Autodesk Inventor part; units mm, degrees
ref_plane "YZ Plane" through (0, 0, 0) normal (1, 0, 0) x (0, 1, 0)
ref_plane "XZ Plane" through (0, 0, 0) normal (0, 1, 0) x (-1, 0, 0)
ref_plane "XY Plane" through (0, 0, 0) normal (0, 0, 1) x (1, 0, 0)
sketch "Sketch1" plane through (0, 0, 0) normal (0, 0, 1) x (1, 0, 0)
  line L0 (-25, -35) -> (25, -35)
  line L1 (30, -30) -> (30, 30)
  line L2 (25, 35) -> (-25, 35)
  line L3 (-30, 30) -> (-30, -30)
  line L4 (-30, -35) -> (30, 35) construction
  line L5 (30, -35) -> (-30, 35) construction
  arc A0 (-25, 35) -> (-30, 30) centre (-25, 30) ccw
  arc A1 (30, 30) -> (25, 35) centre (25, 30) ccw
  arc A2 (25, -35) -> (30, -30) centre (25, -30) ccw
  arc A3 (-30, -30) -> (-25, -35) centre (-25, -30) ccw
  point P0 (0, 0)
  dimension "d0" = 60
  dimension "d1" = 70
  dimension "d4" = 5
extrude "Extrusion1" add sketch "Sketch1" along normal blind 5
sketch "Sketch2" plane through (0, 0, 5) normal (0, 0, 1) x (1, 0, 0)
  line L0 (-22.5, -30.0466) -> (22.5, -30.0466) construction
  line L1 (22.5, -30.0466) -> (22.5, -10.0466) construction
  line L2 (22.5, -10.0466) -> (-22.5, -10.0466) construction
  line L3 (-22.5, -10.0466) -> (-22.5, -30.0466) construction
  line L4 (-22.5, -30.0466) -> (22.5, -10.0466) construction
  line L5 (22.5, -30.0466) -> (-22.5, -10.0466) construction
  point P0 (0, 0)
  point P1 (0, -20.0466)
  point P2 (0, -20.0466)
  dimension "d5" = 45
  dimension "d6" = 20.0466
  dimension "d7" = 20
hole "Hole1" at (22.5, -10.0466, 5) at (22.5, -30.0466, 5) at (-22.5, -30.0466, 5) direction (0, 0, -1) diameter 5.5 depth 8 tip angle 118
sketch "Sketch3" plane through (0, 0, 5) normal (0, 0, 1) x (1, 0, 0)
  line L0 (-2.5, 0) -> (2.5, 0)
  line L1 (2.5, 0) -> (2.5, 20)
  line L2 (2.5, 20) -> (-2.5, 20)
  line L3 (-2.5, 20) -> (-2.5, 0)
  line L4 (-2.5, 0) -> (2.5, 20) construction
  line L5 (2.5, 0) -> (-2.5, 20) construction
  point P0 (0, 0)
  point P1 (0, 10)
  point P2 (0, 10)
  point P3 (0, 0)
  point P4 (0, 10)
  dimension "d15" = 5
  dimension "d16" = 20
  dimension "d17" = 10
extrude "Extrusion2" cut sketch "Sketch3" against normal blind 5
sketch "Sketch4" plane through (0, 0, 5) normal (0, 0, 1) x (1, 0, 0)
  line L0 (-2.5, 20) -> (2.5, 20)
  line L1 (2.5, 0) -> (-2.5, 0)
  point P0 (0, 0)
  point P1 (0, 28)
  point P2 (0, -8)
  point P3 (0, 0)
  dimension "d20" = 8
  dimension "d21" = 8
hole "Hole2" at (0, 28, 5) at (0, -8, 5) direction (0, 0, -1) diameter 4.5 depth 8 tip angle 118
sketch "Sketch5" plane through (0, 0, 5) normal (0, 0, 1) x (1, 0, 0)
  line L0 (2.5, 0) -> (-2.5, 0)
  line L1 (-20, -25) -> (-10, -25)
  line L2 (-10, -25) -> (-10, -20)
  line L3 (-10, -20) -> (-20, -20)
  line L4 (-20, -20) -> (-20, -25)
  line L5 (-20, -25) -> (-10, -20) construction
  line L6 (-10, -25) -> (-20, -20) construction
  line L7 (-25, -35) -> (25, -35)
  line L8 (-30, 30) -> (-30, -30)
  point P0 (0, 0)
  point P1 (0, 0)
  point P2 (-15, -22.5)
  dimension "d34" = 10
  dimension "d35" = 5
  dimension "d36" = 10
  dimension "d37" = 30
  dimension "d38" = 10
extrude "Extrusion3" cut sketch "Sketch5" against normal blind 5
equation "\"d38\" = -0.5 * d34 + 0.5 * d37"
properties part number "Belt_Holder1" material "Polycarbonate, Clear"
Could you check a few things on this model? Use its own coordinates, in mm. A direction names the side the tool comes from. Coordinates: 2 decimals unless noted, no trailing zeros. Write each loop counter-clockwise with the first axis right and the second up, starting at its lowest first coordinate (ties: lowest second). Pieces come first, ordered by that corner, then holes. Notation, with made-up numbers: (1, -10) -> (49, -10) arc R25 ccw to (49, 11) -> close; hole circle Ø9 at (10.25, 77.5). An arc over 180 degrees is marked (long way). One line per question, with ' | ' between items. Start each with the question number.
1. If we section it at D-D (z = 2.1): Please give me the cut outline in (x, y), and give its area (3 significant figures).
2. If we section it at B-B (y = 11): Please give me the cut outline in (x, z).
3. Please list where these lines run through material, in increasing order: line 1 along Y through (x, z) = (0, 1.3); line 2 along Y through (x, z) = (22.5, 2.35); line 3 along X through (y, z) = (3, 2.95).
4. Thinking about a two-plate mould opening in X: for faces 1 (the face through (28, 34, 2)), 2 (the face through (-29, 33, 2)), 3 (the face through (19.773, -9.689, 2.465)), which applies, pulls with the +X half, pulls with the -X half, needs draft (parallel to the pull), parting line crosses it, or undercut?
5. If we section it at A-A (x = 0): Please give me the cut outline in (y, z).
6. For faces 4 (the face through (-30, 0, 2)), 5 (the face through (-10, -23, 3)), which set-ups out of +Z, -Z, +X, -X, +Y, -Y let a thin tool reach every point of the face, with its end or its side?
7. Will this pin go through, and if not, where does the flat tip stop? P1, Ø2.5, axis at x = 0, y = -8, coming from the -Z side.
8. If we section it at C-C (x = 22.5): Please give me the cut outline in (y, z).
Return value:
1) outline: (-30, -30) arc R5 ccw to (-25, -35) -> (25, -35) arc R5 ccw to (30, -30) -> (30, 30) arc R5 ccw to (25, 35) -> (-25, 35) arc R5 ccw to (-30, 30) -> close; hole circle Ø5.5 at (-22.5, -30.05); hole (-20, -25) -> (-10, -25) -> (-10, -20) -> (-20, -20) -> close; hole (-2.5, 0) -> (2.5, 0) -> (2.5, 20) -> (-2.5, 20) -> close; hole circle Ø4.5 at (0, -8); hole circle Ø4.5 at (0, 28); hole circle Ø5.5 at (22.5, -30.05); hole circle Ø5.5 at (22.5, -10.05) | area: 3,930 mm²
2) outline: (-30, 0) -> (-2.5, 0) -> (-2.5, 5) -> (-30, 5) -> close; (2.5, 0) -> (30, 0) -> (30, 5) -> (2.5, 5) -> close
3) line 1: y = -35 to -10.25, -5.75 to 0, 20 to 25.75, 30.25 to 35 | line 2: y = -35 to -32.8, -27.3 to -12.8, -7.3 to 35 | line 3: x = -30 to -2.5, 2.5 to 30
4) face 1: pulls with the +X half | face 2: pulls with the -X half | face 3: undercut
5) outline: (-35, 0) -> (-10.25, 0) -> (-10.25, 5) -> (-35, 5) -> close; (-5.75, 0) -> (0, 0) -> (0, 5) -> (-5.75, 5) -> close; (20, 0) -> (25.75, 0) -> (25.75, 5) -> (20, 5) -> close; (30.25, 0) -> (35, 0) -> (35, 5) -> (30.25, 5) -> close
6) face 4: +Z, -Z, -X, +Y, -Y | face 5: +Z, -Z
7) P1: passes through
8) outline: (-35, 0) -> (-32.8, 0) -> (-32.8, 5) -> (-35, 5) -> close; (-27.3, 0) -> (-12.8, 0) -> (-12.8, 5) -> (-27.3, 5) -> close; (-7.3, 0) -> (35, 0) -> (35, 5) -> (-7.3, 5) -> close
